Autodesk Inventor part; units mm, degrees
ref_plane "Work Plane1" through (-40, 0, 10) normal (0, 1, 0) x (1, 0, 0)
ref_plane "YZ Plane" through (0, 0, 0) normal (1, 0, 0) x (0, 1, 0)
ref_plane "XZ Plane" through (0, 0, 0) normal (0, 1, 0) x (-1, 0, 0)
sketch "Sketch1" plane through (0, 0, 0) normal (0, 0, 1) x (1, 0, 0)
  circle A0 centre (0, 0) radius 70
  dimension "d0" = 140
extrude "Extrusion1" add sketch "Sketch1" along normal blind 10
sketch "Sketch2" plane through (0, 0, 10) normal (0, 0, 1) x (1, 0, 0)
  line L0 (-35, -55) -> (35, -55)
  line L1 (35, -55) -> (35, -35)
  line L2 (35, -35) -> (-35, -35)
  line L3 (-35, -35) -> (-35, -55)
  line L4 (35, 35) -> (-35, 35)
  line L5 (-35, 35) -> (-35, 55)
  line L6 (-35, 55) -> (35, 55)
  line L7 (35, 55) -> (35, 35)
  circle A0 centre (0, 0) radius 70
  line L8 (-35, -35) -> (-60.6218, -35)
  line L9 (35, 35) -> (60.6218, 35)
  line L10 (-35, 35) -> (-60.6218, 35)
  line L11 (35, -35) -> (60.6218, -35)
  dimension "d3" = 35
  dimension "d4" = 35
  dimension "d5" = 20
  dimension "d6" = 70
  dimension "d7" = 35
extrude "Extrusion2" add sketch "Sketch2" along normal blind 155 contours L3 L2 L1 L0 | L5 L6 L7 L4
sketch "Sketch4" plane through (-35, 35, 10) normal (0, -1, 0) x (1, 0, 0)
  line L0 (70, 0) -> (70, 155)
  line L1 (0, 66) -> (70, 66)
  line L2 (70, 66) -> (70, 0)
  line L3 (70, 0) -> (0, 0)
  line L4 (0, 0) -> (0, 66)
  line L5 (0, 66) -> (70, 0) construction
  line L6 (70, 66) -> (0, 0) construction
  circle A0 centre (58.5, 11.5) radius 3
  circle A1 centre (58.5, 58.5) radius 3
  circle A2 centre (11.5, 11.5) radius 3
  circle A3 centre (11.5, 58.5) radius 3
  line L7 (62.5, 62.5) -> (7.5, 62.5)
  line L8 (7.5, 62.5) -> (7.5, 7.5)
  line L9 (7.5, 7.5) -> (62.5, 7.5)
  line L10 (62.5, 7.5) -> (62.5, 62.5)
  circle A4 centre (35, 35) radius 20
  circle A5 centre (35, 35) radius 23
  point P0 (35, -10)
  dimension "d77" = 3
extrude "Extrusion4" add sketch "Sketch4" along normal blind 45 contours L3 L4 L1 L0 | L10 L9 L8 L7
sketch "Sketch3" plane through (-35, 55, 10) normal (0, 1, 0) x (1, 0, 0)
  line L0 (65, -65) -> (5, -65)
  line L1 (5, -65) -> (5, -5)
  line L2 (5, -5) -> (65, -5)
  line L3 (65, -5) -> (65, -65)
  line L4 (-35, 0) -> (105, 0)
  line L5 (70, 0) -> (70, -155)
  line L6 (35, 0) -> (35, -1.4267)
  point P0 (35, 10)
  dimension "d10" = 60
  dimension "d11" = 60
  dimension "d12" = 5
extrude "Extrusion3" cut sketch "Sketch3" against normal blind 60
sketch "Sketch5" plane through (-35, 55, 165) normal (0, 1, 0) x (1, 0, 0)
  circle A0 centre (35, 30) radius 13.5
  line L0 (70, 155) -> (70, 0)
  line L1 (70, 0) -> (0, 0)
  circle A1 centre (35, 30) radius 16.5
  point P0 (35, 165)
  point P1 (70, 125)
  point P2 (70, 69)
  dimension "d28" = 35
  dimension "d29" = 30
  dimension "d40" = 27
  dimension "d84" = 3
extrude "Extrusion5" cut sketch "Sketch5" against normal through all contours A0 | A1
ref_plane "Work Plane2" through (-35, -55, 15) normal (0, -1, 0) x (1, 0, 0)
sketch "Sketch6" plane through (-35, -55, 15) normal (0, -1, 0) x (1, 0, 0)
  circle A0 centre (35, 120) radius 13.5
  circle A1 centre (35, 120) radius 21.5
  circle A2 centre (35, 120) radius 13.5
  point P0 (35, -15)
  dimension "d35" = 8
extrude "Extrusion6" cut sketch "Sketch6" against normal blind 8
ref_plane "Work Plane1" through (-40, 0, 10) normal (0, 1, 0) x (1, 0, 0)
offset faces "Size1" outward -1 faces at (0.663, -35, 46.2068) (-0.663, 35, 90.2068)
fillet "Fillet1" radius 31.5 4 edges at (-35, -45.5, 165) (35, -45.5, 165) (-35, 45.5, 165) (35, 45.5, 165)
sketch "Sketch7" plane through (0, 0, 10) normal (0, 0, 1) x (1, 0, 0)
  circle A0 centre (-50, 25) radius 3
  circle A1 centre (-50, -25) radius 3
  circle A2 centre (50, -25) radius 3
  circle A3 centre (50, 25) radius 3
  circle A4 centre (0, 15) radius 3
  circle A5 centre (0, -15) radius 3
  line L0 (-98, 0) -> (98, 0)
  line L1 (0, 0) -> (0, 59.6277)
  dimension "d41" = 25
  dimension "d42" = 25
  dimension "d43" = 50
  dimension "d44" = 50
  dimension "d45" = 15
  dimension "d46" = 15
  dimension "d47" = 25
  dimension "d48" = 25
  dimension "d49" = 50
  dimension "d50" = 50
  dimension "d51" = 6
extrude "Extrusion7" cut sketch "Sketch7" against normal through all
fillet "Fillet2" radius 5.5 2 edges at (35, 13, 76) (-35, 13, 76)
ref_plane "Work Plane4" through (-35, -55, 15) normal (-1, 0, 0) x (0, 0, 1)
sketch "Sketch8" plane through (-35, -55, 15) normal (-1, 0, 0) x (0, 0, 1)
  line L0 (118.5, 19) -> (118.5, 0)
  line L1 (-5, 19) -> (118.5, 19)
  line L2 (-5, 0) -> (118.5, 0)
  circle A0 centre (73.5, 9.5) radius 2.1
  circle A1 centre (63.5, 9.5) radius 2.1
  line L3 (-5, 0) -> (-5, 19)
  point P0 (-15, 55)
  dimension "d55" = 10
  dimension "d56" = 4.2
  dimension "d57" = 9.5
  dimension "d58" = 45
extrude "Extrusion8" cut sketch "Sketch8" against normal through all contours A0 | A1
chamfer "Chamfer4" distance 8 distance2 48.25 2 edges at (35, -45.5, 10) (-35, -45.5, 10) measured on face at (0.1205, -29.9927, 10)
chamfer "Chamfer5" distance 8 angle 45 2 edges at (35, 22.5, 10) (-35, 22.5, 10)
move faces "Move1" translate (0, 0.5, 0) faces at (0.663, 36, 90.2068)
move faces "Move2" translate (0, -0.5, 0) faces at (0.663, -36, 78.3734)
sketch "Sketch10" plane through (-3.5, 55, 165) normal (0, 1, 0) x (1, 0, 0)
  circle A0 centre (3.5, 30) radius 13.5
  circle A1 centre (3.5, 30) radius 19
  circle A2 centre (3.5, 30) radius 21.5
  circle A3 centre (3.5, 30) radius 15.5
  point P0 (3.5, 165)
  dimension "d73" = 38
  dimension "d74" = 43
  dimension "d83" = 2
extrude "Extrusion9" cut sketch "Sketch10" against normal blind 8 contours A0 | A1 | A2 | A3
sketch "Sketch11" plane through (-35, -55, 58.25) normal (-1, 0, 0) x (0, 0, 1)
  line L0 (0, 18.5) -> (75.25, 18.5)
  line L1 (12.25, 16) -> (12.25, 34.5)
  line L2 (22.25, 16) -> (12.25, 16)
  line L3 (22.25, 34.5) -> (22.25, 16)
  line L4 (12.25, 34.5) -> (22.25, 34.5)
  circle A0 centre (17.25, 25.5) radius 3.2
  line L5 (22.25, 16) -> (12.25, 16)
  line L6 (12.25, 16) -> (12.25, 13)
  line L7 (12.25, 13) -> (22.25, 13)
  line L8 (22.25, 13) -> (22.25, 16)
  line L9 (22.25, 13) -> (23, 13)
  line L10 (23, 13) -> (23, 18.5)
  line L11 (23, 18.5) -> (22.25, 18.5)
  line L12 (22.25, 18.5) -> (22.25, 13)
  line L13 (12.25, 13) -> (11.5, 13)
  line L14 (11.5, 13) -> (11.5, 18.5)
  line L15 (11.5, 18.5) -> (12.25, 18.5)
  line L16 (12.25, 18.5) -> (12.25, 13)
  point P0 (-58.25, 55)
  dimension "d78" = 3
  dimension "d79" = 0.75
  dimension "d80" = 0.75
extrude "Extrusion10" cut sketch "Sketch11" against normal through all contours L0 L1 L6 L13 L14 | L0 L3 L2 L1 | L0 L10 L9 L8 L3 | L2 L8 L7 L6
properties part number "base_3DPrint"
Input: part model. Units: mm. Frame: model coordinates. A direction names the side the tool comes from. Coordinates: 2 decimals unless noted, no trailing zeros. Loops run counter-clockwise (first coordinate to the right, second up) from the corner with the lowest first, then second, coordinate; pieces in that order, holes last.
Q1. Section C-C, the plane x = 0. Give the number of separate pieces and of enclosed holes in the cut face, and give its area (3 significant figures).
Results are:
separate pieces: 5
enclosed holes: 2
area: 4,780 mm2
Q2. Mould query, pull axis Y, two halves, no side actions, for faces 1 (the flat face through (35, -46, 95)), 2 (the flat face through (-1, -55, 69)), 3 (the cylindrical face through (33.43, 12.92, 74.35)). Classes: +Y half, -Y half, draft (parallel to the pull), parting line (faces both ways), or undercut.
Results are:
face 1: draft
face 2: -Y half
face 3: undercut
Q3. Section B-B, the plane y = 25. Return the cut outline in (x, z).
Results are:
outline: (-65.38, 0) - (-53, 0) - (-53, 10) - (-65.38, 10) - close; (-47, 0) - (47, 0) - (47, 10) - (43, 10) - (35, 18) - (35, 70.5) arc R5.5 ccw to (29.5, 76) - (-29.5, 76) arc R5.5 ccw to (-35, 70.5) - (-35, 18) - (-43, 10) - (-47, 10) - close; (53, 0) - (65.38, 0) - (65.38, 10) - (53, 10) - close; hole (-30, 15) - (30, 15) - (30, 75) - (-30, 75) - close
Q4. Section D-D, the plane x = 50. Return the cut outline in (y, z), and give its area (3 significant figures).
Results are:
outline: (-48.99, 0) - (-28, 0) - (-28, 10) - (-48.99, 10) - close; (-22, 0) - (22, 0) - (22, 10) - (-22, 10) - close; (28, 0) - (48.99, 0) - (48.99, 10) - (28, 10) - close
area: 860 mm2
Q5. Contact query for flat-ended pins moving along their axis: pin 1 (23 mm diameter, centred on x = 2.5, y = 20, fed in from +Z); pin 2 (4.5 mm diameter, centred on x = 6, y = -39.5, fed in from +Z); pin 3 (1 mm diameter, centred on x = 34.5, z = 19, fed in from +Y). Output: stop coordinate, or through.
Results are:
pin 1: stops at z = 76
pin 2: stops at z = 165
pin 3: stops at y = 55
Q6. Set-up query: faces 4 (the flat face through (0, 14, 76)), 5 (the cylindrical face through (-2.994, -7.465, 22.196)), 6 (the flat face through (0, 15, 10)). Return all of +Z, -Z, +X, -X, +Y, -Y with unobstructed straight access to the full face (end or side cutting, diameter ignored); none if empty.
Results are:
face 4: +Z, +X, -X
face 5: +Y
face 6: -Z
Q7. Section A-A, the plane z = 78.5. Return the cut outline in (x, y).
Results are:
outline: (-35, -55) - (35, -55) - (35, -47.6) - (-35, -47.6) - close; (-35, -43.4) - (35, -43.4) - (35, -42) - (-35, -42) - close; (-35, 36.5) - (35, 36.5) - (35, 55) - (-35, 55) - close
Q8. Line query: line 1 along X through (y, z) = (-6.5, 68.5); line 2 along Z through (x, y) = (-23.5, -6.2); line 3 along Y through (x, z) = (0, 3). Output: solid intervals per line, ascending.
Results are:
line 1: x = -35 to -26.5, -20.5 to 20.5, 26.5 to 35
line 2: z = 0 to 18.5, 24.5 to 65.5, 71.5 to 76
line 3: y = -70 to -18, -12 to 12, 18 to 70
